Geometry: final body of the model. Coordinates: model frame, mm. A direction names the side the tool comes from. Give positions to 0.01 mm unless a question says otherwise; leave off trailing zeros. Order: outer loops, then holes, each group sorted by start corner. A loop starts at its lowest first (then second) coordinate and runs counter-clockwise, first axis right, second up. Notation, with made-up numbers: (36.5, 76) - (44.5, 76) arc R9 ccw to (44.5, 87) - close; hole circle Ø11 at (77.25, -16). An arc over 180 degrees is marked (long way). Use one line per item in the form item = value.
from build123d import *

# Parameters (mm, degrees)
SKETCH086_R     = 9.35
PAD031_DEPTH    = 20
SKETCH085_R     = 2.25
HOLE033_DEPTH   = 13.001
POCKET034_DEPTH = 3.5
SKETCH087_R     = 2.25
HOLE034_DEPTH   = 8
HOLE034_TIPS_R  = 2.25
POCKET097_DEPTH = 3.4


with BuildPart() as part:
    # Sketch086 → Pad031 (new body)
    with BuildSketch(Plane.XY):
        with BuildLine():
            Line((123.5, 100.5), (123.5, 66))
            ThreePointArc((121.5, 64), (122.914214, 64.585786), (123.5, 66))
            Line((117.5, 64), (121.5, 64))
            ThreePointArc((115.5, 66), (116.085786, 64.585786), (117.5, 64))
            Line((115.5, 95.331912), (115.5, 66))
            ThreePointArc((115.5, 95.331912), (114.625135, 97.828616), (112.383235, 99.233181))
            ThreePointArc((105.51903, 103.01903), (108.683048, 100.640036), (112.383235, 99.233181))
            Line((92.084001, 116.454058), (105.51903, 103.01903))
            Line((101.629942, 126), (92.084001, 116.454058))
            Line((115.5, 126), (101.629942, 126))
            ThreePointArc((128.5, 113), (124.692388, 122.192388), (115.5, 126))
            Line((128.5, 113), (128.5, 109.880832))
            ThreePointArc((124.5, 100.5), (127.458261, 104.781812), (128.5, 109.880832))
            Line((123.5, 100.5), (124.5, 100.5))
        make_face()
        with Locations((115.5, 113)):
            Circle(SKETCH086_R, mode=Mode.SUBTRACT)
    extrude(amount=PAD031_DEPTH)

    # Sketch085 (on DatumPlane) → Hole033 (cut, through all)
    with BuildSketch(Plane.ZY.offset(-115.5)):
        with Locations((10, 90)):
            Circle(SKETCH085_R)
        with Locations((10, 74)):
            Circle(SKETCH085_R)
    extrude(amount=-HOLE033_DEPTH, mode=Mode.SUBTRACT)

    # Sketch084 (on DatumPlane) → Pocket034 (cut)
    with BuildSketch(Plane.ZY.offset(-115.5)):
        Polygon((13.65, 87.892672), (13.65, 92.107328), (10, 94.214657), (6.35, 92.107328), (6.35, 87.892672), (10, 85.785343), align=None)
        Polygon((13.65, 76.107328), (10, 78.214657), (6.35, 76.107328), (6.35, 71.892672), (10, 69.785343), (13.65, 71.892672), align=None)
    extrude(amount=-POCKET034_DEPTH, mode=Mode.SUBTRACT)

    # Sketch087 (on DatumPlane) → Hole034 (cut)
    with BuildSketch(Plane(origin=(-12.185029, 12.185029, 0), x_dir=(-0.707107, -0.707107, 0), z_dir=(-0.707107, 0.707107, 0))):
        with Locations((-154.458676, 5)):
            Circle(SKETCH087_R)
        with Locations((-154.458676, 15)):
            Circle(SKETCH087_R)
    extrude(amount=-HOLE034_DEPTH, mode=Mode.SUBTRACT)

    # Hole034 tips → Hole034 tip 1 section 0
    with BuildSketch(Plane(origin=(-6.528175, 6.528175, 0), x_dir=(-0.707107, -0.707107, 0), z_dir=(-0.707107, 0.707107, 0)), mode=Mode.PRIVATE) as hole034_tip_1_s0:
        with Locations((-154.458676, 5)):
            Circle(HOLE034_TIPS_R)
    loft([hole034_tip_1_s0.sketch, Vertex(103.646566, 114.790988, 5)], mode=Mode.SUBTRACT)

    # Hole034 tips → Hole034 tip 2 section 0
    with BuildSketch(Plane(origin=(-6.528175, 6.528175, 0), x_dir=(-0.707107, -0.707107, 0), z_dir=(-0.707107, 0.707107, 0)), mode=Mode.PRIVATE) as hole034_tip_2_s0:
        with Locations((-154.458676, 15)):
            Circle(HOLE034_TIPS_R)
    loft([hole034_tip_2_s0.sketch, Vertex(103.646566, 114.790988, 15)], mode=Mode.SUBTRACT)

    # Sketch113 (on DatumPlane) → Pocket097 (cut)
    with BuildSketch(Plane(origin=(-10.063708, 10.063708, 0), x_dir=(-0.707107, -0.707107, 0), z_dir=(-0.707107, 0.707107, 0))):
        Polygon((-158.108676, 12.892672), (-154.458676, 10.785343), (-150.808676, 12.892672), (-150.808676, 21), (-158.108676, 21), align=None)
        Polygon((-150.808676, 7.107328), (-154.458676, 9.214657), (-158.108676, 7.107328), (-158.108676, -1), (-150.808676, -1), align=None)
    extrude(amount=-POCKET097_DEPTH, mode=Mode.SUBTRACT)


with BuildPart() as part_1:
    # Body022007 placement: moved
    add(part.part.moved(Location((-2.5, 0, 893))))


solid = part_1.part
(1) Reachability of faces 5 (the face through (113, 81, 903)), 6 (the face through (96.532, 116.789, 901.146)), 7 (the face through (95.259, 115.516, 909.397)), 8 (the face through (95.9, 120.7, 895.8)), 9 (the face through (114.726, 86.824, 904.799)) from +Z, -Z, +X, -X, +Y, -Y: full face, straight path, thin tool, end or side. Return the list, or none.
Computed values:
face_5 = +Z, -Z, -X, -Y
face_6 = -Z
face_7 = +Z
face_8 = none
face_9 = -X
(2) Ray query, line 1 along X through (y, z) = (117.5, 901); line 2 along X through (y, z) = (114.5, 900); line 3 along Y through (x, z) = (118.95, 903). Return the intervals inside material, ascending.
Computed values:
line_1 = 90.63 to 95.46, 99.68 to 104.8, 121.2 to 125.2
line_2 = 91.54 to 96.28, 96.68 to 103.77, 122.23 to 125.91
line_3 = 64 to 71.75, 76.25 to 87.75, 92.25 to 105.79, 120.21 to 124.56
(3) Contact query for flat-ended pins moving along their axis: pin 1 Ø2 at (y, z) = (96.5, 908.5) entering from +X; pin 2 Ø2 at (y, z) = (110.5, 910.5) entering from -X; pin 3 Ø5 at (y, z) = (74, 903) entering from -X. Output: stop coordinate, or through.
Computed values:
pin_1 = 121
pin_2 = 94.54
pin_3 = 116.5
(4) Cut plane B-B on x = 92. Output: boundary loops of the cut face in (y, z), plus the area to 3 significant figures.
Computed values:
outline = (114.04, 893) - (118.87, 893) - (118.87, 913) - (114.04, 913) - close
area = 96.6 mm²
(5) Cut plane C-C on y = 101.5. Output: boundary loops of the cut face in (x, z).
Computed values:
outline = (104.82, 893) - (122.94, 893) - (122.94, 913) - (104.82, 913) - close
(6) Pull-direction query (Y, two-part tool) for faces 1 (the face through (114.726, 93.146, 904.851)), 2 (the face through (94.42, 121.29, 902.86)), 3 (the face through (121, 83, 903)), 4 (the face through (96.21, 109.83, 902.86)); classes: released by +Y, released by -Y, zero draft, split by the parting line, or undercut.
Computed values:
face_1 = undercut
face_2 = released by +Y
face_3 = zero draft
face_4 = released by -Y
(7) Cut plane A-A on y = 74. Output: boundary loops of the cut face in (x, z).
Computed values:
outline = (113, 893) - (121, 893) - (121, 900.75) - (116.5, 900.75) - (116.5, 899.35) - (113, 899.35) - close; (113, 906.65) - (116.5, 906.65) - (116.5, 905.25) - (121, 905.25) - (121, 913) - (113, 913) - close
